Work out the finished part from the listing and answer in its coordinate system (mm). Face numbers are marked on the shaded views. A direction names the side the tool comes from. Round coordinates to 2 decimals unless told otherwise and drop trailing zeros. Order: outer loops, then holes, each group sorted by start corner. A loop starts at its lowest first (then second) coordinate and runs counter-clockwise, first axis right, second up. Notation, with made-up numbers: M 67,-6.5 L 81,-6.5 A7 cw 81,-1.5 Z; hole C -4.75,86 d4. An arc over 180 degrees is marked long. Return JSON: item names as keys, results as strings.
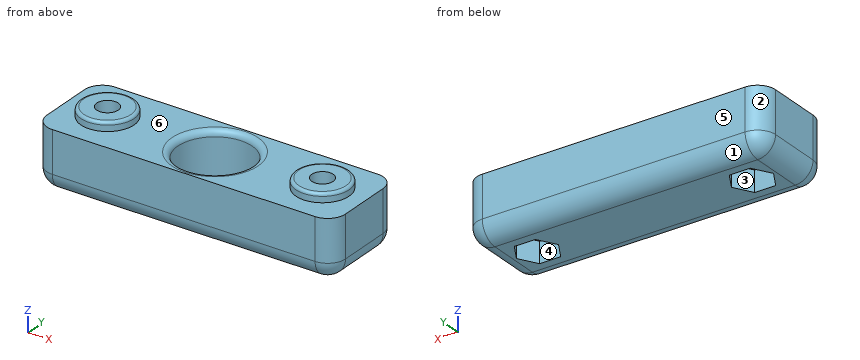
from build123d import *

# Parameters (mm, degrees)
CROQUIS1_W              = 50
CROQUIS1_H              = 15
SALIENTE_EXTRUIR1_DEPTH = 10
CROQUIS2_R              = 6.2
CROQUIS2_R_2            = 4.45
SALIENTE_EXTRUIR2_DEPTH = 1.5
CORTAR_EXTRUIR1_START   = -9.5
CROQUIS3_R              = 6.2
CORTAR_EXTRUIR1_DEPTH   = 9.5
CROQUIS4_R              = 1.8
CORTAR_EXTRUIR2_DEPTH   = 15.5
CORTAR_EXTRUIR3_DEPTH   = 3.5
REDONDEO1_R             = 3
REDONDEO2_R             = 1
REDONDEO3_R             = 0.5


with BuildPart() as part:
    # Croquis1 → Saliente-Extruir1 (new body)
    with BuildSketch(Plane.XY):
        with Locations((-2.430013275, 8.597922849)):
            Rectangle(CROQUIS1_W, CROQUIS1_H)
    extrude(amount=SALIENTE_EXTRUIR1_DEPTH)

    # Croquis2 → Saliente-Extruir2 (add)
    with BuildSketch(Plane.XY.offset(10)):
        with Locations((-2.430013275, 8.597922849)):
            Circle(CROQUIS2_R)
        with Locations((-20.430013275, 8.597922849)):
            Circle(CROQUIS2_R_2)
        with Locations((15.569986725, 8.597922849)):
            Circle(CROQUIS2_R_2)
    extrude(amount=SALIENTE_EXTRUIR2_DEPTH)

    # Croquis3 → Cortar-Extruir1 (cut)
    with BuildSketch(Plane.XY.offset(11.5).offset(CORTAR_EXTRUIR1_START)):
        with Locations((-2.430013275, 8.597922849)):
            Circle(CROQUIS3_R)
    extrude(amount=CORTAR_EXTRUIR1_DEPTH, mode=Mode.SUBTRACT)

    # Croquis4 → Cortar-Extruir2 (cut)
    with BuildSketch(Plane.XY.offset(11.5)):
        with Locations((-20.430013275, 8.597922849)):
            Circle(CROQUIS4_R)
        with Locations((15.569986725, 8.597922849)):
            Circle(CROQUIS4_R)
    extrude(amount=-CORTAR_EXTRUIR2_DEPTH, mode=Mode.SUBTRACT)

    # Croquis5 → Cortar-Extruir3 (cut)
    with BuildSketch(Plane(origin=(0, 0, 0), x_dir=(-1, 0, 0), z_dir=(0, 0, -1))):
        Polygon((-12.048150083, 8.597922849), (-13.809068404, 11.647922849), (-17.330905046, 11.647922849), (-19.091823367, 8.597922849), (-17.330905046, 5.547922849), (-13.809068404, 5.547922849), align=None)
        Polygon((23.951849917, 8.597922849), (22.190931596, 11.647922849), (18.669094954, 11.647922849), (16.908176633, 8.597922849), (18.669094954, 5.547922849), (22.190931596, 5.547922849), align=None)
    extrude(amount=-CORTAR_EXTRUIR3_DEPTH, mode=Mode.SUBTRACT)

    # Redondeo1
    redondeo1_edges = [part.edges().sort_by_distance(p)[0] for p in [
        (-2.430013275, 16.097922849, 0),
        (22.569986725, 8.597922849, 0),
        (-2.430013275, 1.097922849, 0),
        (-27.430013275, 8.597922849, 0),
        (-27.430013275, 16.097922849, 5),
        (22.569986725, 16.097922849, 5),
        (22.569986725, 1.097922849, 5),
        (-27.430013275, 1.097922849, 5),
    ]]
    fillet(redondeo1_edges, radius=REDONDEO1_R)

    # Redondeo2
    redondeo2_edges = [part.edges().sort_by_distance(p)[0] for p in [
        (-8.630013275, 8.597922849, 10),
    ]]
    fillet(redondeo2_edges, radius=REDONDEO2_R)

    # Redondeo3
    redondeo3_edges = [part.edges().sort_by_distance(p)[0] for p in [
        (-24.880013275, 8.597922849, 11.5),
        (11.119986725, 8.597922849, 11.5),
    ]]
    fillet(redondeo3_edges, radius=REDONDEO3_R)


solid = part.part
Item 1: Find section C-C (z = 1). Determine the outline of the cut face in (x, y).
Output:
{"outline": "M -26.67,4.1 A2.24 ccw -24.43,1.86 L 19.57,1.86 A2.24 ccw 21.81,4.1 L 21.81,13.1 A2.24 ccw 19.57,15.33 L -24.43,15.33 A2.24 ccw -26.67,13.1 Z; hole M -23.95,8.6 L -22.19,5.55 L -18.67,5.55 L -16.91,8.6 L -18.67,11.65 L -22.19,11.65 Z; hole M 12.05,8.6 L 13.81,5.55 L 17.33,5.55 L 19.09,8.6 L 17.33,11.65 L 13.81,11.65 Z"}
Item 2: Which of the six approach directions +Z, -Z, +X, -X, +Y, -Y give full straight-line access (tool end or side, diameter ignored) to the marked faces 4, 5 and 6?
Output:
{"face 4": "-Z", "face 5": "+Z, -Z, +X, -X, +Y", "face 6": "+Z"}
Item 3: Find section A-A (z = 6.5). Determine the outline of the cut face in (x, y).
Output:
{"outline": "M -27.43,4.1 A3 ccw -24.43,1.1 L 19.57,1.1 A3 ccw 22.57,4.1 L 22.57,13.1 A3 ccw 19.57,16.1 L -24.43,16.1 A3 ccw -27.43,13.1 Z; hole C -20.43,8.6 d3.6; hole C -2.43,8.6 d12.4; hole C 15.57,8.6 d3.6"}
Item 4: Find section D-D (z = 10.5). Determine the outline of the cut face in (x, y), plus the area to 3 significant figures.
Output:
{"outline": "C -20.43,8.6 d8.9; C 15.57,8.6 d8.9; hole C -20.43,8.6 d3.6; hole C 15.57,8.6 d3.6", "area": "104 mm^2"}
Item 5: Each of these flat-tipped pins is pushed along its axis until it touches: pin 1 (1.5 mm diameter, centred on y = 14, z = 7.5, fed in from -X); pin 2 (6 mm diameter, centred on x = 15.57, y = 8.6, fed in from -Z); pin 3 (1 mm diameter, centred on x = 16, z = 1.5, fed in from -Y); pin 4 (2 mm diameter, centred on x = -20.43, y = 8.6, fed in from +Z). Where does it stop, or does it pass through?
Output:
{"pin 1": "stops at x = -27.43", "pin 2": "stops at z = 3.5", "pin 3": "stops at y = 1.27", "pin 4": "passes through"}
Item 6: The mould has two halves that part along X. Classify the marked faces 1, 2 and 3: pulls with the +X half, pulls with the -X half, needs draft (parallel to the pull), parting line crosses it, or undercut.
Output:
{"face 1": "needs draft", "face 2": "pulls with the -X half", "face 3": "undercut"}
Item 7: Find section B-B (x = 10). Determine the outline of the cut face in (y, z).
Output:
{"outline": "M 1.1,3 A3 ccw 4.1,0 L 13.1,0 A3 ccw 16.1,3 L 16.1,10 L 1.1,10 Z"}
Item 8: Consider line 1 along X through (y, z) = (7.75, 9); line 2 along X through (y, z) = (7.75, 9.75); line 3 along Z through (x, y) = (-14, 4). Determine where each line is inside the solid, lowest interval first. Write a range as [from, to].
Output:
{"line 1": "x = [-27.43, -22.02], [-18.84, -8.57], [3.71, 13.98], [17.16, 22.57]", "line 2": "x = [-27.43, -22.02], [-18.84, -8.91], [4.05, 13.98], [17.16, 22.57]", "line 3": "z = [0, 10]"}
